Input: part model. Units: mm. Frame: model coordinates. Face numbers are marked on the shaded views. Coordinates: 2 decimals unless noted, no trailing zeros. Loops run counter-clockwise (first coordinate to the right, second up) from the corner with the lowest first, then second, coordinate; pieces in that order, holes last. Notation, with made-up numbers: (8, 20) - (40, 20) arc R6 ccw to (40, 27) - close; hole circle Ø10 at (7.5, 22). An arc over 180 degrees is marked (long way). Use a Markdown table: item, result. Add a question column.
1. Ray query, L1, parallel to X at y = 80, z = -30; L2, parallel to Y at x = -13, z = -21.5; L3, parallel to Y at x = -19.05, z = -13. Return the intervals inside material, ascending. Write a range as [from, to].
2. Draft query along Y for the marked faces 1, 2 and 3. Return one class per face: released by +Y, released by -Y, zero draft, split by the parting line, or undercut.
3. Section query C-C on x = -15. Return the cut outline in (y, z) (1 decimal), then the cut area to 3 significant figures.
4. Section query B-B on x = -6. Return the cut outline in (y, z) (1 decimal).
5. Section query D-D on x = -25. Return the cut outline in (y, z) (3 decimals).
6. Section query A-A on y = 80. Return the cut outline in (x, z) (1 decimal), then the cut area to 3 significant figures.
7. Contact query for a flat-ended pin moving along its axis: P1, Ø5, axis at x = -16.5, z = -19, coming from the -Y side. Output: stop coordinate, or through.
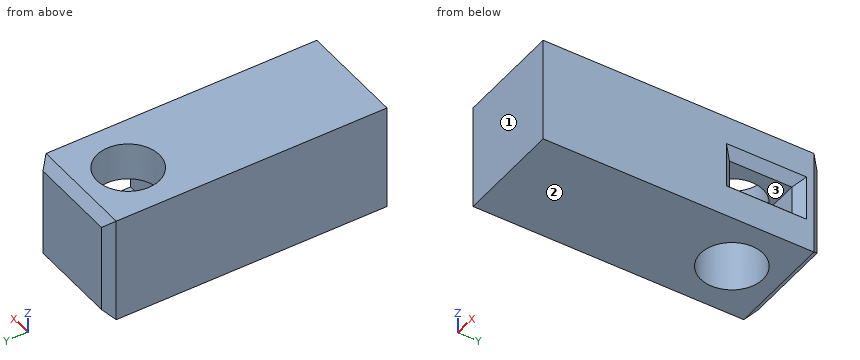
Autodesk Inventor part; units mm, degrees
ref_plane "YZ Plane" through (0, 0, 0) normal (1, 0, 0) x (0, 1, 0)
ref_plane "XZ Plane" through (0, 0, 0) normal (0, 1, 0) x (-1, 0, 0)
ref_plane "XY Plane" through (0, 0, 0) normal (0, 0, 1) x (1, 0, 0)
sketch "Sketch1" plane through (0, 0, 0) normal (0, 1, 0) x (-1, 0, 0)
  line L0 (0, 0) -> (38.1, 0)
  line L1 (38.1, 0) -> (38.1, -38.1)
  line L2 (38.1, -38.1) -> (0, -38.1)
  line L3 (0, -38.1) -> (0, 0)
  dimension "d0" = 38.1
  dimension "d1" = 38.1
extrude "Extrusion1" add sketch "Sketch1" along normal blind 100
sketch "Sketch2" plane through (0, 0, -38.1) normal (0, 0, -1) x (-1, 0, 0)
  circle A0 centre (19.05, 80) radius 11.15
  line L0 (0, 100) -> (38.1, 100)
  line L1 (0, 0) -> (0, 100)
  dimension "d4" = 22.3
  dimension "d5" = 20
  dimension "d6" = 19.05
sketch "Sketch3" plane through (0, 0, -38.1) normal (0, 0, -1) x (-1, 0, 0)
  point P0 (0, 0)
extrude "Extrusion2" cut sketch "Sketch2" against normal blind 38.1
sketch "Sketch4" plane through (0, 0, 0) normal (1, 0, 0) x (0, 0, -1)
  line L0 (13.4535, 68.7) -> (23.4535, 68.7)
  line L1 (23.4535, 68.7) -> (23.4535, 91)
  line L2 (23.4535, 91) -> (13.4535, 91)
  line L3 (13.4535, 91) -> (13.4535, 68.7)
  line L4 (13.4535, 68.7) -> (23.4535, 91) construction
  line L5 (23.4535, 68.7) -> (13.4535, 91) construction
  line L6 (0, 100) -> (38.1, 100)
  point P0 (0, 0)
  point P1 (18.4535, 79.85)
  dimension "d9" = 10
  dimension "d10" = 22.3
  dimension "d11" = 9
extrude "Extrusion3" cut sketch "Sketch4" against normal blind 19.05
chamfer "Chamfer1" distance 3.175 angle 45 8 edges at (0, 91, -18.4535) (0, 68.7, -18.4535) (0, 79.85, -13.4535) (0, 79.85, -23.4535) (0, 100, -19.05) (-19.05, 100, -38.1) (-38.1, 100, -19.05) (-19.05, 100, 0)
properties part number "XTower"
Resolved:
| question | item | result |
|---|---|---|
| 1 | L1 | [-38.1, -30.2], [-7.9, 0] |
| 1 | L2 | [0, 68.7], [91, 100] |
| 1 | L3 | [0, 68.85], [91.15, 100] |
| 2 | face 1 | released by -Y |
| 2 | face 2 | zero draft |
| 2 | face 3 | undercut |
| 3 | outline | (0, -38.1) - (69.6, -38.1) - (69.6, -23.5) - (68.7, -23.5) - (68.7, -13.5) - (69.6, -13.5) - (69.6, 0) - (0, 0) - close; (90.4, -38.1) - (96.8, -38.1) - (100, -34.9) - (100, -3.2) - (96.8, 0) - (90.4, 0) - (90.4, -13.5) - (91, -13.5) - (91, -23.5) - (90.4, -23.5) - close |
| 3 | area | 2,990 mm² |
| 4 | outline | (0, -38.1) - (96.8, -38.1) - (100, -34.9) - (100, -3.2) - (96.8, 0) - (0, 0) - close; hole (68.7, -23.5) - (91, -23.5) - (91, -13.5) - (68.7, -13.5) - close |
| 5 | outline | (0, -38.1) - (70.57, -38.1) - (70.57, 0) - (0, 0) - close; (89.43, -38.1) - (96.825, -38.1) - (100, -34.925) - (100, -3.175) - (96.825, 0) - (89.43, 0) - close |
| 6 | outline | (-38.1, -38.1) - (-30.2, -38.1) - (-30.2, 0) - (-38.1, 0) - close; (-7.9, -38.1) - (0, -38.1) - (0, -26.6) - (-3.2, -23.5) - (-7.9, -23.5) - close; (-7.9, -13.5) - (-3.2, -13.5) - (0, -10.3) - (0, 0) - (-7.9, 0) - close |
| 6 | area | 513 mm² |
| 7 | P1 | y = 0 |
